Design review of the part built by this model. Coordinates are the model's own, in mm. Give positions to 0.01 mm unless a question says otherwise; leave off trailing zeros. Write each loop counter-clockwise with the first axis right and the second up, starting at its lowest first coordinate (ties: lowest second). Pieces come first, ordered by that corner, then holes. Notation, with made-up numbers: M -20,42 L 15,42 A22 ccw 15,57 Z; hole C -15,43 d8. An arc over 180 degrees is marked long. Answer in a Markdown table with one row per item.
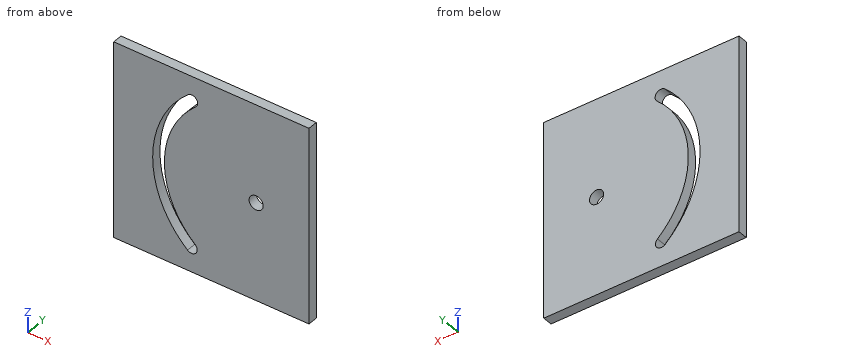
```python
from build123d import *

# Parameters (mm, degrees)
F0_W     = 200
F0_H     = 200
F0_R     = 7.25
F1_DEPTH = 10


with BuildPart() as f1:
    # F0 (on Front) → F1 (new body)
    with BuildSketch(Plane.XZ):
        Rectangle(F0_W, F0_H)
        with BuildLine():
            ThreePointArc((-24.4348083961, -79.4901646735), (-60.1255414788, 0.098775478), (-24.0407608064, 79.5098353265))
            ThreePointArc((-24.0407608064, 79.5098353265), (-15.5734786606, 78.9574468193), (-16.1258671678, 70.4901646735))
            ThreePointArc((-16.1258671678, 70.4901646735), (-48.12557833, 0.0690361286), (-16.4753055963, -70.5098353265))
            ThreePointArc((-16.4753055963, -70.5098353265), (-15.9648923227, -78.9797513999), (-24.4348083961, -79.4901646735))
        make_face(mode=Mode.SUBTRACT)
        with Locations((45.8741330018, -0.1639221083)):
            Circle(F0_R, mode=Mode.SUBTRACT)
    extrude(amount=F1_DEPTH)


solid = f1.part
```
1) Add section C-C (y = -4.25). Write out the cut boundary in (x, z).
Geometry says:
| item | result |
|---|---|
| outline | M -100,-100 L 100,-100 L 100,100 L -100,100 Z; hole M -24.43,-79.49 A6 ccw -16.48,-70.51 A94 cw -16.13,70.49 A6 ccw -24.04,79.51 A106 ccw Z; hole C 45.87,-0.16 d14.5 |
2) Add section A-A (z = -46). Write out the cut boundary in (x, y).
Geometry says:
| item | result |
|---|---|
| outline | M -100,-10 L -49.7,-10 L -49.7,0 L -100,0 Z; M -36.19,-10 L 100,-10 L 100,0 L -36.19,0 Z |
3) Add section B-B (x = -53). Write out the cut boundary in (y, z).
Geometry says:
| item | result |
|---|---|
| outline | M -10,-100 L 0,-100 L 0,-38.37 L -10,-38.37 Z; M -10,38.04 L 0,38.04 L 0,100 L -10,100 Z |
4) Insertion check: P1, Ø12, axis at x = -65.5, z = -15.5, coming from the +Y side. The pin has a flat end and moves straight along its axis. Give the tip position at first contact, or say it passes through.
Geometry says:
| item | result |
|---|---|
| P1 | y = 0 |
5) To check wall thickness, follow probe 1 along X at (y, z) = (-7.25, -61); probe 2 along X at (y, z) = (-3.75, -19); probe 3 along Z at (x, y) = (51.5, -3.5). State the ranges of each line that lie inside material, in increasing order. Write a range as [from, to].
Geometry says:
| item | result |
|---|---|
| probe 1 | [-100, -40.93], [-25.78, 100] |
| probe 2 | [-100, -58.44], [-46.22, 100] |
| probe 3 | [-100, -4.74], [4.41, 100] |
